```python
from build123d import *

# Parameters (mm, degrees)
F0_W          = 105
F0_H          = 145
F1_DEPTH      = 71
F2_T          = -2.5
F3_W          = 1
F3_H          = 29
F4_DEPTH      = 62
F5_W          = 50
F5_H          = 1.5
F6_DEPTH      = 142.5
F6_DEPTH_BACK = 268
F7_R          = 1


# Not quite as in the source:
# - an extrude ends at something that could not be found from the text; its depth is read off the source's solid


with BuildPart() as f1:
    # F0 (on Top) → F1 (new body)
    with BuildSketch(Plane.XY):
        Rectangle(F0_W, F0_H)
    extrude(amount=F1_DEPTH)

    # F2
    f2_openings = [f1.faces().sort_by_distance(p)[0] for p in [
        (0, 0, 71),
    ]]
    offset(amount=F2_T, openings=f2_openings)

    # F3 (on face) → F4 (join)
    with BuildSketch(Plane.XY.offset(2.5)):
        Polygon((-50, -40), (-50, -41), (-0.5, -41), (0.5, -41), (50, -41), (50, -40), align=None)
        with Locations((0, -55.5)):
            Rectangle(F3_W, F3_H)
    extrude(amount=F4_DEPTH)

    # F5 (on face) → F6 (cut, two sides)
    with BuildSketch(Plane.XZ.offset(72.5)) as f6_sk:
        with Locations((25, 70.25)):
            Rectangle(F5_W, F5_H)
        with Locations((-25, 70.25)):
            Rectangle(F5_W, F5_H)
        Polygon((50, 69.5), (0, 69.5), (0, 68), (51.2, 68), align=None)
        Polygon((0, 68), (0, 69.5), (-50, 69.5), (-51.2, 68), align=None)
    extrude(amount=-F6_DEPTH, mode=Mode.SUBTRACT)
    extrude(f6_sk.sketch, amount=F6_DEPTH_BACK, mode=Mode.SUBTRACT)

    # F7
    f7_edges = [f1.edges().sort_by_distance(p)[0] for p in [
        (52.5, -72.5, 35.5),
        (52.5, 72.5, 35.5),
        (52.5, 0, 0),
        (52.5, 0, 71),
        (-52.5, 72.5, 35.5),
        (-52.5, -72.5, 35.5),
        (-52.5, 0, 0),
        (-52.5, 0, 71),
        (0, 72.5, 0),
        (0, 72.5, 71),
        (0, -72.5, 0),
        (-51.25, -72.5, 71),
        (51.25, -72.5, 71),
    ]]
    fillet(f7_edges, radius=F7_R)


solid = f1.part
```
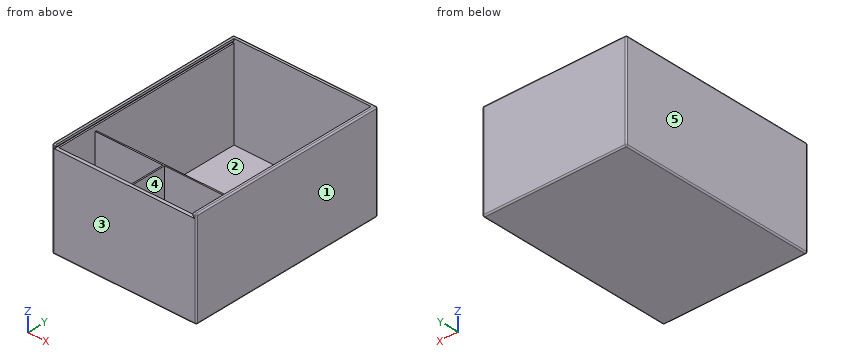
Could you check a few things on this model? Use its own coordinates, in mm. Face numbers are marked on the shaded views. A direction names the side the tool comes from. Give positions to 0.01 mm unless a question says otherwise; leave off trailing zeros. Write each loop counter-clockwise with the first axis right and the second up, starting at its lowest first coordinate (ties: lowest second). Pieces come first, ordered by that corner, then holes. Notation, with made-up numbers: (1, 46.25) -> (8, 46.25) arc R35 cw to (8, 82.25) -> close; hole circle Ø4 at (-35, -7). An arc over 180 degrees is marked (long way). Write each question's results on one line, items separated by ' | '.
1. If we mould it in two halves opening along Y, with no side actions, what happens to the marked faces 3, 4 and 5? For each: released by +Y, released by -Y, zero draft, split by the parting line, or undercut.
Check sheet entries:
face 3: released by -Y | face 4: undercut | face 5: zero draft
2. On a 3-axis mill with a long thin cutter (end or side, diameter ignored), from which of +Z, -Z, +X, -X, +Y, -Y can I reach the whole of each face in a straight line? I mean the marked faces 1 and 2. Say none if no direction works.
Check sheet entries:
face 1: +Z, -Z, +X, +Y, -Y | face 2: +Z
3. I want a section at D-D, the plane y = -18.5. Write out the boundary of the cut face in (x, z), then the cut area to 3 significant figures.
Check sheet entries:
outline: (-52.5, 1) arc R1 ccw to (-51.5, 0) -> (51.5, 0) arc R1 ccw to (52.5, 1) -> (52.5, 70) arc R1 ccw to (51.5, 71) -> (50, 71) -> (50, 69.5) -> (51.2, 68) -> (50, 68) -> (50, 2.5) -> (-50, 2.5) -> (-50, 68) -> (-51.2, 68) -> (-50, 69.5) -> (-50, 71) -> (-51.5, 71) arc R1 ccw to (-52.5, 70) -> close | area: 602 mm²
4. Will this pin go through, and if not, where does the flat tip stop? pin 1 Ø1 at (x, y) = (-27.5, 48) entering from +Z.
Check sheet entries:
pin 1: stops at z = 2.5
5. I want a section at B-B, the plane y = -48. Write out the boundary of the cut face in (x, z), then the cut area to 3 significant figures.
Check sheet entries:
outline: (-52.5, 1) arc R1 ccw to (-51.5, 0) -> (51.5, 0) arc R1 ccw to (52.5, 1) -> (52.5, 70) arc R1 ccw to (51.5, 71) -> (50, 71) -> (50, 69.5) -> (51.2, 68) -> (50, 68) -> (50, 2.5) -> (0.5, 2.5) -> (0.5, 64.5) -> (-0.5, 64.5) -> (-0.5, 2.5) -> (-50, 2.5) -> (-50, 68) -> (-51.2, 68) -> (-50, 69.5) -> (-50, 71) -> (-51.5, 71) arc R1 ccw to (-52.5, 70) -> close | area: 664 mm²
6. I need wall thicknesses on L1, parallel to Y at x = 30, z = 13; L2, parallel to X at y = -53.5, z = 23; L3, parallel to X at y = 5, z = 20.5. Which ranges of each line are inside material? Lowest first, please.
Check sheet entries:
L1: y = -72.5 to -70, -41 to -40, 70 to 72.5 | L2: x = -52.5 to -50, -0.5 to 0.5, 50 to 52.5 | L3: x = -52.5 to -50, 50 to 52.5
7. I want a section at C-C, the plane x = -42. Write out the boundary of the cut face in (y, z).
Check sheet entries:
outline: (-72.5, 1) arc R1 ccw to (-71.5, 0) -> (71.5, 0) arc R1 ccw to (72.5, 1) -> (72.5, 70) arc R1 ccw to (71.5, 71) -> (70, 71) -> (70, 2.5) -> (-40, 2.5) -> (-40, 64.5) -> (-41, 64.5) -> (-41, 2.5) -> (-70, 2.5) -> (-70, 68) -> (-72.5, 68) -> close
8. I want a section at A-A, the plane z = 40. Write out the boundary of the cut face in (x, y).
Check sheet entries:
outline: (-52.5, -71.5) arc R1 ccw to (-51.5, -72.5) -> (51.5, -72.5) arc R1 ccw to (52.5, -71.5) -> (52.5, 71.5) arc R1 ccw to (51.5, 72.5) -> (-51.5, 72.5) arc R1 ccw to (-52.5, 71.5) -> close; hole (-50, -70) -> (-0.5, -70) -> (-0.5, -41) -> (-50, -41) -> close; hole (-50, -40) -> (50, -40) -> (50, 70) -> (-50, 70) -> close; hole (0.5, -70) -> (50, -70) -> (50, -41) -> (0.5, -41) -> close
